from build123d import *

# Parameters (mm, degrees)
F0_R     = 4
F1_DEPTH = 6
F3_SIZE  = 0.4
F4_R     = 0.1


# Not quite as in the source:
# - a fillet or chamfer that OpenCascade refuses, or shapes differently, is made with other operations: its cross-section is extruded or revolved along the edge and cut away or added


with BuildPart() as f1:
    # F0 (on Top) → F1 (new body)
    with BuildSketch(Plane.XY):
        Circle(F0_R)
    extrude(amount=F1_DEPTH)

    # F2: chamfer of 0.2 x 11.4579923262 on 1 edges, made by hand

    # F2_s1 → F2_t2 (revolve, cut)
    with BuildSketch(Plane.XZ):
        Polygon((4, -5.4579923262), (3.8, 6), (4, 6), align=None)
    revolve(axis=Axis((0, 0, 6), (0, 0, 1)), mode=Mode.SUBTRACT)

    # F3
    f3_edges = [f1.edges().sort_by_distance(p)[0] for p in [
        (-3.8, 0, 6),
    ]]
    chamfer(f3_edges, length=F3_SIZE)

    # F4
    f4_edges = [f1.edges().sort_by_distance(p)[0] for p in [
        (-3.4, 0, 6),
        (-3.806981, 0, 5.600061),
    ]]
    fillet(f4_edges, radius=F4_R)


solid = f1.part
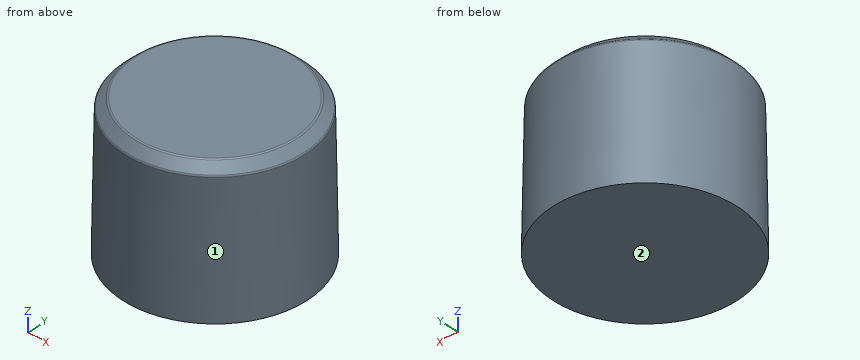
For this review, take the finished solid that the model builds, in its own axes (mm). Face numbers are marked on the shaded views. A direction names the side the tool comes from. Round coordinates to 2 decimals unless told otherwise and drop trailing zeros. Order: outer loops, then holes, each group sorted by start corner. A loop starts at its lowest first (then second) coordinate and runs counter-clockwise, first axis right, second up. Notation, with made-up numbers: (9, -12) -> (15, -12) arc R32 cw to (15, 21) -> close; hole circle Ø7 at (-8.5, 28.5). An arc over 180 degrees is marked (long way). Write item = value, one per line. Start each with the question number.
1) Tool access review of the marked faces 1 and 2: name each direction out of +Z, -Z, +X, -X, +Y, -Y from which nothing blocks a thin tool from reaching the whole face with its end or side.
2) Insertion check: pin 1 (3 mm diameter, centred on x = 2.5, y = 3, fed in from -Z). The pin has a flat end and moves straight along its axis. Give the tip position at first contact, or say it passes through.
3) Take a section at A-A on z = 2.5. State the section outline as (x, y) points.
4) To check wall thickness, follow line 1 (Y direction, x = -0.5, z = 3.75); line 2 (Z direction, x = -2, y = 3); line 3 (Y direction, x = 2.5, z = 1). State the ranges of each line that lie inside material, in increasing order. Write a range as from..to.
5) Take a section at B-B on z = 4. State the section outline as (x, y) points.
Verdict:
q1.face_1 = +Z
q1.face_2 = -Z, +X, -X, +Y, -Y
q2.pin_1 = 0
q3.outline = circle Ø7.72 at (0, 0)
q4.line_1 = -3.81..3.81
q4.line_2 = 0..5.8
q4.line_3 = -2.98..2.98
q5.outline = circle Ø7.67 at (0, 0)
